Geometry: final body of the model. Coordinates: model frame, mm. Face numbers are marked on the shaded views. A direction names the side the tool comes from. Coordinates: 2 decimals unless noted, no trailing zeros. Loops run counter-clockwise (first coordinate to the right, second up) from the corner with the lowest first, then second, coordinate; pieces in that order, holes last. Notation, with made-up numbers: (31, 76) -> (51, 76) arc R27 cw to (51, 108) -> close; hole circle Ø3 at (25, 89). An arc over 180 degrees is marked (long way). One line per item, written item: value. Start each with the question number.
Item 1: Section query A-A on z = -84. Return loops of the section in (x, y), then the cut area to 3 significant figures.
Item 2: Section query D-D on x = 16. Return loops of the section in (y, z), then the cut area to 3 significant figures.
Item 3: Section query C-C on z = -50.5. Return loops of the section in (x, y) (3 decimals), then the cut area to 3 significant figures.
Item 4: Section query B-B on x = 50. Return loops of the section in (y, z).
Item 5: Ray query, probe 1 along Z at (x, y) = (71, 7.75); probe 2 along Z at (x, y) = (70, 4.25); probe 3 along X at (y, z) = (6.25, -36) (3 decimals). Return the intervals inside material, ascending. Write a range as from..to.
Item 6: Contact query for flat-ended pins moving along their axis: pin 1 Ø3 at (x, z) = (32, -52) entering from -Y; pin 2 Ø1.1 at (x, y) = (90.5, 4.5) entering from -Z; pin 3 Ø1.5 at (y, z) = (4, -19) entering from +X. Output: stop coordinate, or through.
Item 7: Mould query, pull axis Z, two halves, no side actions, for the marked faces 3 and 4. Classes: +Z half, -Z half, draft (parallel to the pull), parting line (faces both ways), or undercut.
Item 8: Set-up query: the marked faces 1 and 2. Return all of +Z, -Z, +X, -X, +Y, -Y with unobstructed straight access to the full face (end or side cutting, diameter ignored); none if empty.
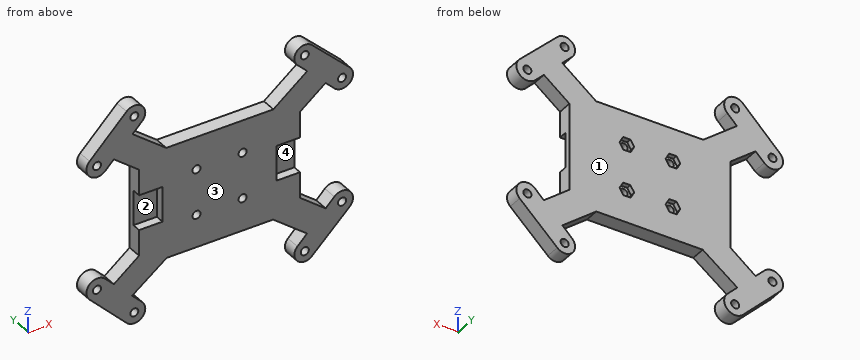
Autodesk Inventor part; units mm, degrees
ref_plane "Work Plane1" through (0, 1.6, 0) normal (0, 1, 0) x (1, 0, 0)
ref_plane "YZ Plane" through (0, 0, 0) normal (1, 0, 0) x (0, 1, 0)
ref_plane "XZ Plane" through (0, 0, 0) normal (0, 1, 0) x (-1, 0, 0)
ref_plane "Work Plane1" through (0, 1.6, 0) normal (0, 1, 0) x (1, 0, 0)
sketch "Sketch2" plane through (0, 1.6, 0) normal (0, 1, 0) x (1, 0, 0)
  circle A0 centre (23, 7) radius 1.75
  line L0 (21.25, 7) -> (23, 7)
  circle A1 centre (6.8172, 22.8502) radius 1.75
  line L1 (5.0672, 22.8502) -> (6.8172, 22.8502)
  circle A2 centre (6.8172, 77.1499) radius 1.75
  line L2 (5.0672, 77.1499) -> (6.8172, 77.1499)
  circle A3 centre (23, 93) radius 1.75
  line L3 (21.25, 93) -> (23, 93)
  circle A4 centre (97, 7) radius 1.75
  line L4 (95.25, 7) -> (97, 7)
  circle A5 centre (113.1829, 22.8502) radius 1.75
  line L5 (111.4329, 22.8502) -> (113.1829, 22.8502)
  circle A6 centre (113.1829, 77.1499) radius 1.75
  line L6 (111.4329, 77.1499) -> (113.1829, 77.1499)
  circle A7 centre (97, 93) radius 1.75
  line L7 (95.25, 93) -> (97, 93)
  circle A8 centre (23, 7) radius 1.75
  circle A9 centre (6.8172, 22.8502) radius 1.75
  circle A10 centre (6.8172, 77.1499) radius 1.75
  circle A11 centre (23, 93) radius 1.75
  circle A12 centre (97, 93) radius 1.75
  circle A13 centre (113.1829, 77.1499) radius 1.75
  circle A14 centre (113.1829, 22.8502) radius 1.75
  circle A15 centre (97, 7) radius 1.75
  line L8 (6.8172, 22.8502) -> (2.2899, 22.8502)
  line L9 (6.8172, 22.8502) -> (3.6159, 19.6489)
  line L10 (23, 7) -> (18.2375, 7)
  line L11 (23, 7) -> (19.6324, 3.6324)
  line L12 (19.6324, 3.6324) -> (3.6159, 19.6489)
  line L13 (6.8172, 22.8502) -> (10.3511, 26.3841)
  line L14 (23, 7) -> (26.3676, 10.3676)
  line L15 (120, 100.0001) -> (0, 100.0001)
  line L16 (113.1829, 77.1499) -> (108.4204, 77.1499)
  line L17 (113.1829, 77.1499) -> (109.8153, 73.7823)
  line L18 (113.1829, 77.1499) -> (116.5505, 80.5175)
  line L19 (97, 93) -> (92.4727, 93)
  line L20 (97, 93) -> (93.7987, 89.7988)
  line L21 (97, 93) -> (100.2013, 96.2013)
  line L22 (116.5505, 80.5175) -> (100.2013, 96.2013)
  line L23 (23, 7) -> (6.8172, 22.8502)
  line L24 (23, 7) -> (23, -11.3324)
  line L25 (23, 7) -> (14.9089, 14.9248)
  line L26 (113.1829, 77.1499) -> (97, 93)
  line L27 (97, 93) -> (97, 106.2617)
  line L28 (97, 93) -> (105.0911, 85.0752)
  line L29 (0, 0) -> (0, 50)
  line L30 (0, 100.0001) -> (0, 0)
  line L31 (120, 0) -> (120, 100.0001)
  line L32 (19.6324, 96.3676) -> (3.6159, 80.3511)
  line L33 (116.5505, 19.4826) -> (100.2013, 3.7987)
  arc A16 (19.6324, 3.6324) -> (26.3676, 10.3676) centre (23, 7) ccw
  arc A17 (10.3511, 26.3841) -> (3.6159, 19.6489) centre (6.9835, 23.0165) ccw
  line L34 (22.0621, 85.327) -> (37.0786, 74.1625)
  line L35 (83.2604, 74.1625) -> (97.9859, 85.6116)
  arc A18 (3.6159, 80.3511) -> (10.3511, 73.6159) centre (6.9835, 76.9835) ccw
  arc A19 (26.3676, 89.6324) -> (19.6324, 96.3676) centre (23, 93) ccw
  arc A20 (116.5505, 19.4826) -> (109.8153, 26.2178) centre (113.1829, 22.8502) ccw
  line L36 (93.7987, 10.2013) -> (98.0654, 14.3802)
  line L37 (106.0172, 22.4978) -> (109.8153, 26.2178)
  arc A21 (109.8153, 73.7823) -> (116.5505, 80.5175) centre (113.1829, 77.1499) ccw
  arc A22 (100.2013, 96.2013) -> (93.7987, 89.7988) centre (97, 93) ccw
  line L38 (10.3511, 73.6159) -> (14.1298, 77.3946)
  line L39 (22.0621, 85.327) -> (26.3676, 89.6324)
  arc A23 (93.7987, 10.2013) -> (100.2013, 3.7987) centre (97, 7) ccw
  line L40 (15.5072, 21.228) -> (10.3511, 26.3841)
  line L41 (26.3676, 10.3676) -> (22.2406, 14.4946)
  line L42 (109.8153, 73.7823) -> (106.0611, 77.5364)
  line L43 (97.9859, 85.6116) -> (93.7987, 89.7988)
  line L44 (22.2406, 14.4946) -> (15.5072, 21.228)
  line L45 (6.8172, 22.8502) -> (6.8172, 36.0698)
  line L46 (31.9559, 119.5066) -> (31.9559, 155.0666)
  line L47 (31.9559, 155.0666) -> (-39.1641, 155.0666)
  line L48 (-39.1641, 155.0666) -> (-39.1641, 119.5066)
  line L49 (-39.1641, 119.5066) -> (31.9559, 119.5066)
  line L50 (24.3041, 175.988) -> (54.7841, 175.988)
  line L51 (54.7841, 175.988) -> (54.7841, 203.928)
  line L52 (54.7841, 203.928) -> (24.3041, 203.928)
  line L53 (24.3041, 203.928) -> (24.3041, 175.988)
  line L54 (83.3672, 25.8376) -> (36.8534, 25.8376)
  line L55 (83.2604, 74.1625) -> (37.0786, 74.1625)
  line L56 (94.925, 31.1303) -> (94.925, 68.8698)
  line L57 (22.2406, 14.4946) -> (36.8534, 25.8376)
  line L58 (98.0654, 14.3802) -> (83.3672, 25.8376)
  line L59 (0, 50) -> (34.6, 50)
  line L60 (103.7116, 86.4264) -> (120, 100.0001)
  line L61 (106.0611, 77.5364) -> (94.925, 68.8698)
  line L62 (34.6, 50) -> (109.6103, 50)
  line L63 (14.1298, 77.3946) -> (25.075, 68.8698)
  line L64 (106.0611, 22.4637) -> (94.925, 31.1303)
  line L65 (14.1298, 22.6054) -> (25.075, 31.1303)
  line L66 (25.075, 68.8698) -> (25.075, 31.1303)
  dimension "d20" = 45
  dimension "d21" = 45
  dimension "d22" = 45
  dimension "d23" = 45
  dimension "d26" = 50
  dimension "d41" = 16.0165
  dimension "d42" = 4.7625
  dimension "d43" = 4.7625
  dimension "d44" = 6.7335
  dimension "d45" = 134.405
  dimension "d49" = 71.12
  dimension "d50" = 35.56
  dimension "d53" = 27.94
  dimension "d54" = 30.48
extrude "Extrusion4" add sketch "Sketch2" along normal blind 6.35 contours A0 L14 A16 L24 | A0 L23 A1 L13 L40 L44 L41 L14 | L24 A16 L11 A0 | A0 L11 L12 L9 A1 L23 | L44 L40 L65 L66 L59 L62 L56 L64 L37 A20 L33 A23 L36 L58 L54 L57 | A17 L45 A1 L9 | A17 L13 A1 L45 | L66 L63 L38 A18 L32 A19 L39 L34 L55 L35 L43 L20 A7 L26 A6 L17 L42 L61 L56 L62 L59 | A22 L21 A7 L27 | L27 A7 L19 A22 | L60 L26 A7 L21 L22 | L22 L18 A6 L26 L60 | L19 A7 L20 A22 | L17 A6 L18 A21
sketch "Sketch18" plane through (0, 1.6, 0) normal (0, -1, 0) x (1, 0, 0)
  line L0 (83.2604, -74.1625) -> (37.0786, -74.1625)
  line L1 (22.2406, -14.4946) -> (36.8534, -25.8376)
  line L2 (94.925, -74.1625) -> (25.075, -74.1625)
  line L3 (25.075, -74.1625) -> (25.075, -25.8376)
  line L4 (25.075, -25.8376) -> (94.925, -25.8376)
  line L5 (94.925, -25.8376) -> (94.925, -74.1625)
  line L6 (75, -66) -> (45, -66)
  line L7 (45, -66) -> (45, -34.0001)
  line L8 (45, -34.0001) -> (75, -34.0001)
  line L9 (75, -34.0001) -> (75, -66)
  line L10 (70, -60) -> (50, -60)
  line L11 (50, -60) -> (50, -40)
  line L12 (50, -40) -> (70, -40)
  line L13 (70, -40) -> (70, -60)
  line L14 (0, -99.1742) -> (0, 0)
  circle A0 centre (50, -60) radius 1.75
  circle A1 centre (50, -40) radius 1.75
  circle A2 centre (70, -60) radius 1.75
  circle A3 centre (70, -40) radius 1.75
  point P0 (94.925, -71.2652)
  point P1 (25.075, -28.6863)
  dimension "d111" = 29.9999
  dimension "d112" = 48.3249
  dimension "d113" = 69.85
  dimension "d114" = 31.9999
  dimension "d115" = 19.925
  dimension "d118" = 20
  dimension "d119" = 20
  dimension "d120" = 5
  dimension "d121" = 25.075
  dimension "d122" = 6
  dimension "d124" = 3.5
  dimension "d125" = 3.5
  dimension "d126" = 3.5
  dimension "d127" = 3.5
  dimension "d130" = 8.1625
extrude "Extrusion15" cut sketch "Sketch18" against normal blind 12.9499 contours A0 L11 L10 | L10 L11 A0 | A2 L13 L10 | L10 L13 A2 | A1 L12 L11 | L11 L12 A1 | A3 L12 L13 | L13 L12 A3
sketch "Sketch25" plane through (0, 7.95, 0) normal (0, 1, 0) x (1, 0, 0)
  circle A0 centre (70, 40) radius 1.75
  line L0 (70, 40) -> (66.826, 39.9225)
  line L1 (70, 40) -> (68.3459, 42.7101)
  line L2 (70, 40) -> (71.5199, 42.7876)
  line L3 (70, 40) -> (73.1741, 40.0775)
  line L4 (70, 40) -> (71.6542, 37.29)
  line L5 (70, 40) -> (68.4801, 37.2125)
  line L6 (73.1741, 40.0775) -> (71.5199, 42.7876)
  line L7 (71.5199, 42.7876) -> (68.3459, 42.7101)
  line L8 (66.826, 39.9225) -> (68.3459, 42.7101)
  line L9 (68.4801, 37.2125) -> (66.826, 39.9225)
  line L10 (71.6542, 37.29) -> (73.1741, 40.0775)
  line L11 (71.6542, 37.29) -> (68.4801, 37.2125)
  line L12 (70, 60) -> (66.826, 59.9225)
  line L13 (70, 60) -> (68.3459, 62.7101)
  line L14 (70, 60) -> (71.5199, 62.7876)
  line L15 (70, 60) -> (73.1741, 60.0775)
  line L16 (70, 60) -> (71.6542, 57.29)
  line L17 (70, 60) -> (68.4801, 57.2125)
  line L18 (73.1741, 60.0775) -> (71.5199, 62.7876)
  line L19 (71.5199, 62.7876) -> (68.3459, 62.7101)
  line L20 (66.826, 59.9225) -> (68.3459, 62.7101)
  line L21 (68.4801, 57.2125) -> (66.826, 59.9225)
  line L22 (71.6542, 57.29) -> (73.1741, 60.0775)
  line L23 (71.6542, 57.29) -> (68.4801, 57.2125)
  line L24 (50, 60) -> (46.8259, 59.9225)
  line L25 (50, 60) -> (48.3459, 62.7101)
  line L26 (50, 60) -> (51.5199, 62.7876)
  line L27 (50, 60) -> (53.1741, 60.0775)
  line L28 (50, 60) -> (51.6542, 57.29)
  line L29 (50, 60) -> (48.4801, 57.2125)
  line L30 (53.1741, 60.0775) -> (51.5199, 62.7876)
  line L31 (51.5199, 62.7876) -> (48.3459, 62.7101)
  line L32 (46.8259, 59.9225) -> (48.3459, 62.7101)
  line L33 (48.4801, 57.2125) -> (46.8259, 59.9225)
  line L34 (51.6542, 57.29) -> (53.1741, 60.0775)
  line L35 (51.6542, 57.29) -> (48.4801, 57.2125)
  line L36 (50, 40) -> (46.8259, 39.9225)
  line L37 (50, 40) -> (48.3459, 42.7101)
  line L38 (50, 40) -> (51.5199, 42.7876)
  line L39 (50, 40) -> (53.1741, 40.0775)
  line L40 (50, 40) -> (51.6542, 37.29)
  line L41 (50, 40) -> (48.4801, 37.2125)
  line L42 (53.1741, 40.0775) -> (51.5199, 42.7876)
  line L43 (51.5199, 42.7876) -> (48.3459, 42.7101)
  line L44 (46.8259, 39.9225) -> (48.3459, 42.7101)
  line L45 (48.4801, 37.2125) -> (46.8259, 39.9225)
  line L46 (51.6542, 37.29) -> (53.1741, 40.0775)
  line L47 (51.6542, 37.29) -> (48.4801, 37.2125)
  circle A1 centre (70, 60) radius 1.75
  line L48 (70, 60) -> (70, 63.9973)
  circle A2 centre (50, 60) radius 1.75
  line L49 (50, 60) -> (50, 63.553)
  circle A3 centre (50, 40) radius 1.75
  line L50 (50, 40) -> (49.9075, 43.787)
  point P0 (0, 0)
  dimension "d241" = 34.925
  dimension "d244" = 15.2456
  dimension "d245" = 10.16
  dimension "d168" = 3.175
  dimension "d169" = 3.175
  dimension "d170" = 3.175
  dimension "d171" = 3.175
  dimension "d172" = 3.175
  dimension "d173" = 3.175
  dimension "d174" = 60
  dimension "d175" = 60
  dimension "d176" = 60
  dimension "d177" = 60
  dimension "d178" = 60
  dimension "d179" = 3.175
  dimension "d180" = 3.175
  dimension "d181" = 3.175
  dimension "d182" = 3.175
  dimension "d183" = 3.175
  dimension "d184" = 3.175
  dimension "d185" = 60
  dimension "d186" = 60
  dimension "d187" = 60
  dimension "d188" = 60
  dimension "d189" = 60
  dimension "d190" = 3.175
  dimension "d191" = 3.175
  dimension "d192" = 3.175
  dimension "d193" = 3.175
  dimension "d194" = 3.175
  dimension "d195" = 3.175
  dimension "d196" = 60
  dimension "d197" = 60
  dimension "d198" = 60
  dimension "d199" = 60
  dimension "d200" = 60
  dimension "d201" = 3.175
  dimension "d202" = 3.175
  dimension "d203" = 3.175
  dimension "d204" = 3.175
  dimension "d205" = 3.175
  dimension "d206" = 3.175
  dimension "d207" = 60
  dimension "d208" = 60
  dimension "d209" = 60
  dimension "d210" = 60
  dimension "d211" = 60
extrude "Extrusion22" cut sketch "Sketch25" against normal blind 2.159 contours A0 L3 L10 L4 | A0 L2 L6 L3 | L4 L11 L5 A0 | A0 L1 L7 L2 | L5 L9 L0 A0 | A0 L0 L8 L1 | A1 L17 L21 L12 | L12 L20 L13 A1 | L13 L19 L48 A1 | A1 L48 L19 L14 | L14 L18 L15 A1 | L15 L22 L16 A1 | L16 L23 L17 A1 | A2 L29 L33 L24 | L24 L32 L25 A2 | L25 L31 L49 A2 | A2 L49 L31 L26 | L26 L30 L27 A2 | L27 L34 L28 A2 | L28 L35 L29 A2 | A3 L41 L45 L36 | L36 L44 L37 A3 | L37 L43 L50 A3 | A3 L50 L43 L38 | L38 L42 L39 A3 | L39 L46 L40 A3 | L40 L47 L41 A3
sketch "Sketch30" plane through (0, 1.6, 0) normal (0, -1, 0) x (1, 0, 0)
  line L0 (36.8534, -25.8376) -> (83.3672, -25.8376)
  line L1 (36.8534, -25.8376) -> (26.6397, -25.8376)
  line L2 (26.6397, -25.8376) -> (19.1384, -25.8376)
  line L3 (25.075, -28.6863) -> (15.5072, -21.228)
  line L4 (25.075, -28.6863) -> (25.075, -19.9564)
  line L5 (25.075, -71.2738) -> (25.075, -28.6863)
  line L6 (25.075, -71.2738) -> (25.075, -79.7824)
  line L7 (83.2604, -74.1625) -> (37.0786, -74.1625)
  line L8 (37.0786, -74.1625) -> (22.4586, -74.1625)
  line L9 (25.075, -25.8376) -> (35.235, -25.8376)
  line L10 (35.235, -25.8376) -> (35.235, -74.1625)
  line L11 (35.235, -74.1625) -> (25.075, -74.1625)
  line L12 (25.075, -74.1625) -> (25.075, -25.8376)
  line L13 (25.075, -25.8376) -> (25.075, -50.0057)
  line L14 (25.075, -50.0057) -> (35.235, -50)
  line L15 (35.235, -50) -> (35.235, -42.38)
  line L16 (25.075, -50.0057) -> (25.075, -57.6257)
  line L17 (35.235, -42.38) -> (25.075, -42.38)
  line L18 (25.075, -42.38) -> (25.075, -57.6257)
  line L19 (25.075, -57.6257) -> (35.235, -57.6257)
  line L20 (35.235, -57.6257) -> (35.235, -42.38)
  line L21 (83.3672, -25.8376) -> (97.0518, -25.8376)
  line L22 (94.925, -28.7897) -> (94.925, -24.641)
  line L23 (94.925, -25.8376) -> (60, -25.8376)
  line L24 (60, -25.8376) -> (60, -91.5414)
  line L25 (94.925, -25.8376) -> (94.925, -50.0057)
  line L26 (94.925, -50.0057) -> (94.925, -57.6257)
  line L27 (84.765, -42.38) -> (94.925, -42.38)
  line L28 (94.925, -57.6257) -> (84.765, -57.6257)
  line L29 (84.765, -57.6257) -> (84.765, -42.38)
  point P0 (0, 0)
  dimension "d235" = 10.16
  dimension "d236" = 24.1681
  dimension "d237" = 7.62
  dimension "d238" = 7.62
  dimension "d241" = 34.925
  dimension "d244" = 15.2456
  dimension "d245" = 10.16
extrude "Extrusion30" cut sketch "Sketch30" against normal blind 3.81 contours L25 L26 L28 L29 L27 | L10 L14 L5 L17 | L10 L19 L5 L14
properties part number "Drone_cross"
Reply:
1. outline: (7.26, 1.6) -> (23.85, 1.6) -> (23.85, 7.95) -> (7.26, 7.95) -> close; (95.91, 1.6) -> (112.92, 1.6) -> (112.92, 7.95) -> (95.91, 7.95) -> close
1. area: 213 mm²
2. outline: (1.6, -92.74) -> (7.95, -92.74) -> (7.95, -75.94) -> (1.6, -75.94) -> close; (1.6, -24.06) -> (7.95, -24.06) -> (7.95, -7.26) -> (1.6, -7.26) -> close
2. area: 213 mm²
3. outline: (25.075, 5.41) -> (35.235, 5.41) -> (35.235, 1.6) -> (84.765, 1.6) -> (84.765, 5.41) -> (94.925, 5.41) -> (94.925, 7.95) -> (25.075, 7.95) -> close
3. area: 366 mm²
4. outline: (1.6, -74.16) -> (7.95, -74.16) -> (7.95, -62.75) -> (5.79, -62.75) -> (5.79, -61.75) -> (1.6, -61.75) -> close; (1.6, -58.25) -> (5.79, -58.25) -> (5.79, -57.25) -> (7.95, -57.25) -> (7.95, -42.75) -> (5.79, -42.75) -> (5.79, -41.75) -> (1.6, -41.75) -> close; (1.6, -38.25) -> (5.79, -38.25) -> (5.79, -37.25) -> (7.95, -37.25) -> (7.95, -25.84) -> (1.6, -25.84) -> close
5. probe 1: z = -74.16..-62.77, -57.27..-42.77, -37.27..-25.84
5. probe 2: z = -74.16..-61.75, -58.25..-41.75, -38.25..-25.84
5. probe 3: x = 25.075..94.925
6. pin 1: stops at y = 5.41
6. pin 2: stops at z = -80.22
6. pin 3: stops at x = 116.8
7. face 3: draft
7. face 4: undercut
8. face 1: +Z, -Z, +X, -X, +Y
8. face 2: -X, -Y
